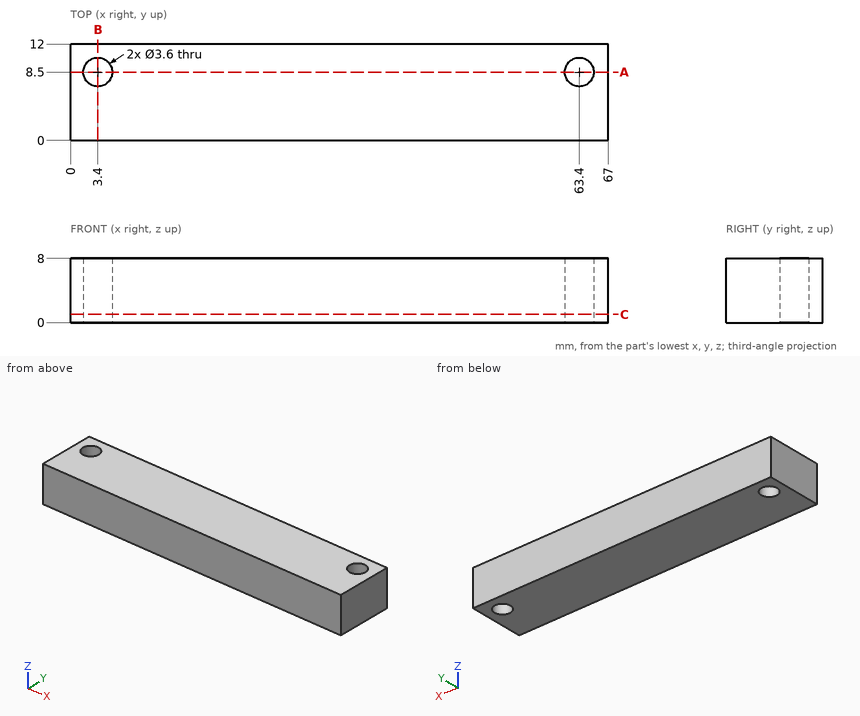
The drawing under review shows one solid part. Ordinate dimensions are in mm from its lowest x, y, z. Round coordinates to 2 decimals unless told otherwise and drop trailing zeros. Write each loop counter-clockwise with the first axis right and the second up, starting at its lowest first coordinate (ties: lowest second). Pieces come first, ordered by that corner, then holes. Notation, with made-up numbers: M 39,77 L 97,77 A9 cw 97,93 Z; hole C 57,30.5 d1. An arc over 180 degrees is marked long. One line per item, written item: value. Start each with the question number.
(1) Wall thickness on line 1 (Y direction, x = 3.4, z = 3); line 2 (X direction, y = 9, z = 0.5); line 3 (X direction, y = 9.25, z = 3): over which ranges is each line inside the solid? List them lowest first.
(2) We need section A-A (y = 8.5). Give the boundary of the cut face in (x, z), and give its area (3 significant figures).
(3) We need section C-C (z = 1). Give the boundary of the cut face in (x, y).
(4) We need section B-B (x = 3.4). Give the boundary of the cut face in (y, z), and give its area (3 significant figures).
Result:
1. line 1: 0 to 6.7, 10.3 to 12
1. line 2: 0 to 1.67, 5.13 to 61.67, 65.13 to 67
1. line 3: 0 to 1.76, 5.04 to 61.76, 65.04 to 67
2. outline: M 0,0 L 1.6,0 L 1.6,8 L 0,8 Z; M 5.2,0 L 61.6,0 L 61.6,8 L 5.2,8 Z; M 65.2,0 L 67,0 L 67,8 L 65.2,8 Z
2. area: 478 mm²
3. outline: M 0,0 L 67,0 L 67,12 L 0,12 Z; hole C 3.4,8.5 d3.6; hole C 63.4,8.5 d3.6
4. outline: M 0,0 L 6.7,0 L 6.7,8 L 0,8 Z; M 10.3,0 L 12,0 L 12,8 L 10.3,8 Z
4. area: 67.2 mm²
